Read the model definition and answer for the solid it produces. Units are mm, in the model's axes. A direction names the side the tool comes from. Round coordinates to 2 decimals unless told otherwise and drop trailing zeros. Order: outer loops, then holes, each group sorted by start corner. A loop starts at its lowest first (then second) coordinate and runs counter-clockwise, first axis right, second up. Notation, with made-up numbers: (-36.5, 58.25) -> (-12.5, 58.25) arc R19 cw to (-12.5, 70.25) -> close; hole circle Ø3 at (45, 37). An arc over 180 degrees is marked (long way). Answer as a JSON object with one key per item and string values. Group by question number.
Item 1: Section B-B, the plane y = -3 is taken. Write down the section's boundary in (x, z).
Item 2: Given P1, Ø8, axis at y = -0.5, z = 73, coming from the -X side; P2, Ø1.6, axis at x = -35, y = 2.5, coming from the +Z side; P3, Ø0.6, axis at x = -35.5, y = 3, coming from the -Z side, each flat-ended and moving along its own axis, determine where each tip first touches the part or whether it passes through.
Item 3: The mould has two halves that part along Z. Classify faces 4 (the flat face through (24.54, 7.54, 36.8)), 5 (the flat face through (-35, 0, 46)), 6 (the flat face through (33.5, 5, 44)), 7 (the cylindrical face through (-11.82, 7.535, 14.887)): pulls with the +Z half, pulls with the -Z half, needs draft (parallel to the pull), parting line crosses it, or undercut.
Item 4: Section A-A, the plane z = 52 is taken. Write down the section's boundary in (x, y).
Item 5: Section C-C, the plane z = 35.5 is taken. Write down the section's boundary in (x, y).
Item 6: Consider probe 1 along X at (y, z) = (8, -2.5); probe 2 along Z at (x, y) = (-28.5, 7.25); probe 3 along Z at (x, y) = (29, 4). Determine where each line is inside the solid, lowest interval first. Write a range as from..to.
Item 7: Section D-D, the plane z = -11 is taken. Write down the section's boundary in (x, y), plus the area to 3 significant figures.
Item 8: For faces 1 (the flat face through (0, 5, 2.5)), 2 (the flat face through (-30.44, 0.94, 88.3)), 3 (the flat face through (0, 2, -5)), determine the directions among +Z, -Z, +X, -X, +Y, -Y from which every point of the face is accessible in a straight line to the end or side of a thin tool.
from build123d import *

# Parameters (mm, degrees)
BOSS_EXTRUDE1_DEPTH = 10
FILLET2_R           = 30
SKETCH6_R           = 1
BOSS_EXTRUDE2_DEPTH = 5
SKETCH4_W           = 2
SKETCH4_H           = 1.5
CUT_EXTRUDE1_DEPTH  = 99.900202224
FILLET3_R           = 15
CUT_REVOLVE1_START  = -1
CUT_REVOLVE1_DEPTH  = 3.5
FILLET1_R           = 10
FILLET4_R           = 1
FILLET5_R           = 2
BOSS_EXTRUDE3_START = -10
BOSS_EXTRUDE3_DEPTH = 15
DELETEFACE1_DEPTH   = 11
FILLET6_R           = 3
FILLET7_R           = 3
BOSS_EXTRUDE4_START = -10
SKETCH11_W          = 10
SKETCH11_H          = 0.3
BOSS_EXTRUDE4_DEPTH = 8
FILLET8_R           = 0.3


with BuildPart() as part:
    # Sketch2 → Boss-Extrude1 (new body)
    with BuildSketch(Plane(origin=(0, 0, 0), x_dir=(1, 0, 0), z_dir=(0, 1, 0))):
        with BuildLine():
            Line((-15, 2.5), (-15, -2.5))
            Line((-15, -2.5), (15, -2.5))
            Line((15, -2.5), (15, 2.5))
            Line((15, 2.5), (-12, 2.5))
            ThreePointArc((-12, 2.5), (-36.874067112, 16.717067208), (-36.5, -11.93086969))
            Line((-36.5, -11.93086969), (-36.5, -66.907529531))
            ThreePointArc((-36.5, -66.907529531), (-34.28320825, -78.052094241), (-27.970319449, -87.5))
            Line((-27.970319449, -87.5), (-25.848999105, -85.378679656))
            ThreePointArc((-25.848999105, -85.378679656), (-31.511569653, -76.904043944), (-33.5, -66.907529531))
            Line((-33.5, -66.907529531), (-33.5, -10.039936204))
            ThreePointArc((-33.5, -10.039936204), (-36.074628704, 13.674748319), (-15, 2.5))
        make_face()
    boss_extrude1 = extrude(amount=BOSS_EXTRUDE1_DEPTH)

    # Mirror2: Boss-Extrude1 across plane
    add(boss_extrude1.mirror(Plane(origin=(0, 0, 0), x_dir=(0, 0, 1), z_dir=(1, 0, 0))))

    # Fillet2
    fillet2_edges = [part.edges().sort_by_distance(p)[0] for p in [
        (-36.5, 5, 11.93086969),
        (36.5, 5, 11.93086969),
    ]]
    fillet(fillet2_edges, radius=FILLET2_R)

    # Sketch6 → Boss-Extrude2 (add)
    # profile 1 of 2: a face of its own
    with BuildSketch(Plane(origin=(0, 10, 0), x_dir=(1, 0, 0), z_dir=(0, 1, 0))):
        with BuildLine():
            Line((-32.29175747, -29.0937848), (-16.524124365, -17.1403988))
            ThreePointArc((-16.524124365, -17.1403988), (-11.748018495, -14.869514069), (-6.462616651, -14.688870483))
            ThreePointArc((-6.462616651, -14.688870483), (-4.151991915, -13.057609213), (-5.783253184, -10.746984477))
            ThreePointArc((-5.783253184, -10.746984477), (-12.694932518, -10.983210705), (-18.940609425, -13.9528292))
            Line((-18.940609425, -13.9528292), (-34.70824253, -25.9062152))
            ThreePointArc((-34.70824253, -25.9062152), (-35.0937848, -28.70824253), (-32.29175747, -29.0937848))
        make_face()
        with Locations(Location((-6.122934918, -12.71792748, 0), (0, 0, 270))):
            Circle(SKETCH6_R, mode=Mode.SUBTRACT)
    # profile 2 of 2: a face of its own
    with BuildSketch(Plane(origin=(0, 10, 0), x_dir=(1, 0, 0), z_dir=(0, 1, 0))):
        with BuildLine():
            Line((32.29175747, -25.9062152), (16.524124365, -37.8596012))
            ThreePointArc((16.524124365, -37.8596012), (11.748018495, -40.130485931), (6.462616651, -40.311129517))
            ThreePointArc((6.462616651, -40.311129517), (4.151991915, -41.942390787), (5.783253184, -44.253015523))
            ThreePointArc((5.783253184, -44.253015523), (12.694932518, -44.016789295), (18.940609425, -41.0471708))
            Line((18.940609425, -41.0471708), (34.70824253, -29.0937848))
            ThreePointArc((34.70824253, -29.0937848), (35.0937848, -26.29175747), (32.29175747, -25.9062152))
        make_face()
        with Locations(Location((6.122934918, -42.28207252, 0), (0, 0, 270))):
            Circle(SKETCH6_R, mode=Mode.SUBTRACT)
    extrude(amount=-BOSS_EXTRUDE2_DEPTH)

    # Sketch4 → Cut-Extrude1 (cut, through all)
    with BuildSketch(Plane(origin=(0, 10, 0), x_dir=(1, 0, 0), z_dir=(0, 1, 0))):
        with BuildLine():
            Line((-13.2, 2.5), (-13.2, -2.5))
            Line((-13.2, -2.5), (-14.040055325, -2.5))
            ThreePointArc((-14.040055325, -2.5), (-43.588524672, 5.0350391), (-13.2, 2.5))
        make_face()
        with Locations((-35.5, -59.25)):
            Rectangle(SKETCH4_W, SKETCH4_H)
        with Locations((-35.5, -62.75)):
            Rectangle(SKETCH4_W, SKETCH4_H)
        with Locations((-35.5, -55.75)):
            Rectangle(SKETCH4_W, SKETCH4_H)
        with Locations((-35.5, -66.25)):
            Rectangle(SKETCH4_W, SKETCH4_H)
        with Locations((-35.5, -69.75)):
            Rectangle(SKETCH4_W, SKETCH4_H)
        with Locations((35.5, -69.75)):
            Rectangle(SKETCH4_W, SKETCH4_H)
        with Locations((35.5, -66.25)):
            Rectangle(SKETCH4_W, SKETCH4_H)
        with Locations((35.5, -62.75)):
            Rectangle(SKETCH4_W, SKETCH4_H)
        with Locations((35.5, -55.75)):
            Rectangle(SKETCH4_W, SKETCH4_H)
        with Locations((35.5, -59.25)):
            Rectangle(SKETCH4_W, SKETCH4_H)
        with BuildLine():
            Line((13.2, -2.5), (14.040055325, -2.5))
            ThreePointArc((14.040055325, -2.5), (43.588524672, 5.0350391), (13.2, 2.5))
            Line((13.2, 2.5), (13.2, -2.5))
        make_face()
    extrude(amount=-CUT_EXTRUDE1_DEPTH, mode=Mode.SUBTRACT)

    # Fillet3
    fillet3_edges = [part.edges().sort_by_distance(p)[0] for p in [
        (33.5, 5, 11.959944675),
        (-33.5, 5, 11.959944675),
    ]]
    fillet(fillet3_edges, radius=FILLET3_R)

    # Cut-Revolve1: read off the stored shape, not the designer's step
    # Cut-Revolve1 outline → Cut-Revolve1 (cut)
    with BuildSketch(Plane(origin=(0, 0, 0), x_dir=(1, 0, 0), z_dir=(0, 1, 0)).offset(CUT_REVOLVE1_START)):
        with BuildLine():
            ThreePointArc((-41.983870968, -7.00974362), (-39.626617248, -9.683939782), (-36.75, -11.789419162))
            Line((-36.75, -11.789419162), (-36.469117037, -11.3029156))
            ThreePointArc((-36.469117037, -11.3029156), (-37.473434742, -10.092280811), (-38.599009901, -8.993476368))
            ThreePointArc((-38.599009901, -8.993476368), (-34.807739235, 16.439240501), (-13.2, 2.5))
            Line((-13.2, 2.5), (-12, 2.5))
            ThreePointArc((-12, 2.5), (-33.488292745, 18.227903086), (-41.983870968, -7.00974362))
        make_face()
    cut_revolve1 = extrude(amount=CUT_REVOLVE1_DEPTH, mode=Mode.SUBTRACT)

    # Mirror3: Cut-Revolve1 across plane
    add(cut_revolve1.mirror(Plane(origin=(0, 0, 0), x_dir=(0, 0, 1), z_dir=(1, 0, 0))), mode=Mode.SUBTRACT)

    # Fillet1
    fillet1_edges = [part.edges().sort_by_distance(p)[0] for p in [
        (-12, 6.25, -2.5),
        (12, 6.25, -2.5),
    ]]
    fillet(fillet1_edges, radius=FILLET1_R)

    # Fillet4
    # the kernel refuses this fillet: 1 mm, written as the material it takes off along each edge
    with BuildSketch(Plane(origin=(41.983870968, -16.048184468, 7.00974362), x_dir=(-0.7225326531123375, 0, 0.6913367957706624), z_dir=(0, 1, 0))) as fillet4_piece_1:
        with BuildLine():
            CenterArc((6.528208905, 0.981393724), FILLET4_R, 113.353303502, 145.576812808)
            ThreePointArc((6.131809124, 1.899471723), (3.116855905, 0.785256492), (0, 0))
            ThreePointArc((0, 0), (3.168101381, 0.307003562), (6.336202761, 0))
        make_face()
    extrude(amount=18.548184468, mode=Mode.SUBTRACT)
    with BuildSketch(Plane(origin=(-41.983870968, -16.048184468, 7.00974362), x_dir=(0.7225326531123378, 0, 0.6913367957706622), z_dir=(0, 1, 0))) as fillet4_piece_2:
        with BuildLine():
            CenterArc((6.528208905, -0.981393724), FILLET4_R, 101.06988369, 145.576812808)
            ThreePointArc((6.131809124, -1.899471723), (3.116855905, -0.785256492), (0, 0))
            ThreePointArc((0, 0), (3.168101381, -0.307003562), (6.336202761, 0))
        make_face()
    extrude(amount=18.548184468, mode=Mode.SUBTRACT)

    # Fillet5
    fillet5_edges = [part.edges().sort_by_distance(p)[0] for p in [
        (-33.5, 7.5, 29.5),
        (-33.5, 7.5, 24.99025088),
        (33.5, 7.5, 25.5),
        (33.5, 7.5, 30.00974912),
    ]]
    fillet(fillet5_edges, radius=FILLET5_R)

    # Sketch8 → Boss-Extrude3 (add)
    with BuildSketch(Plane.XZ.offset(BOSS_EXTRUDE3_START)):
        with BuildLine():
            Line((-26.213914484, 95.605099549), (-31.869667291, 94.247080891))
            Line((-31.869667291, 94.247080891), (-27.783825698, 77.230738791))
            Line((-27.783825698, 77.230738791), (-22.128072891, 78.588757448))
            ThreePointArc((-22.128072891, 78.588757448), (-26.909659277, 86.439339828), (-26.213914484, 95.605099549))
        make_face()
    boss_extrude3 = extrude(amount=BOSS_EXTRUDE3_DEPTH)

    # Mirror4: Boss-Extrude3 across plane
    add(boss_extrude3.mirror(Plane(origin=(0, 0, 0), x_dir=(0, 0, 1), z_dir=(1, 0, 0))))

    # DeleteFace1: read off the stored shape, not the designer's step
    # DeleteFace1 outline → DeleteFace1 (cut)
    with BuildSketch(Plane(origin=(0, 0, 0), x_dir=(1, 0, 0), z_dir=(0, 1, 0))):
        with BuildLine():
            Line((25.848999105, -85.378679656), (26.909659277, -86.439339828))
            ThreePointArc((26.909659277, -86.439339828), (26.685366049, -85.610488056), (26.414012779, -84.795828548))
            ThreePointArc((26.414012779, -84.795828548), (26.133770133, -85.089449001), (25.848999105, -85.378679656))
        make_face()
        with BuildLine():
            Line((-26.909659277, -86.439339828), (-25.848999105, -85.378679656))
            ThreePointArc((-25.848999105, -85.378679656), (-26.133770133, -85.089449001), (-26.414012779, -84.795828548))
            ThreePointArc((-26.414012779, -84.795828548), (-26.685366049, -85.610488056), (-26.909659277, -86.439339828))
        make_face()
    extrude(amount=DELETEFACE1_DEPTH, mode=Mode.SUBTRACT)

    # Fillet6
    fillet6_edges = [part.edges().sort_by_distance(p)[0] for p in [
        (-31.869667291, 2.5, 94.247080891),
        (-29.774582906, 5, 85.521663663),
        (-27.783825698, 2.5, 77.230738791),
        (29.774582906, 5, 85.521663663),
        (27.783825698, 2.5, 77.230738791),
        (31.869667291, 2.5, 94.247080891),
    ]]
    fillet(fillet6_edges, radius=FILLET6_R)

    # Fillet7
    # the kernel refuses this fillet: 3 mm, written as the material it adds along each edge
    with BuildSketch(Plane(origin=(28.870158832, 10, 81.755000397), x_dir=(-0.4451552484524621, 0, -0.8954534073726151), z_dir=(0, -1, 0))) as fillet7_piece_1:
        with BuildLine():
            CenterArc((5.429938119, 2.554031947), FILLET7_R, 138.932760823, 99.425389741)
            Line((3.168120681, 4.524864735), (2.941938938, 4.721948013))
            ThreePointArc((2.941938938, 4.721948013), (1.218371107, 2.518472645), (-0.262566045, 0.145117443))
            Line((-0.262566045, 0.145117443), (0.067135427, -0.292391577))
            ThreePointArc((0.067135427, -0.292391577), (1.678072021, 0.077492249), (3.698732127, -0.255403195))
            Line((3.698732127, -0.255403195), (3.85611449, 0))
        make_face()
    extrude(amount=10)
    with BuildSketch(Plane(origin=(-28.870158832, 10, 81.755000397), x_dir=(-0.47821106545327013, 0, -0.8782449412766623), z_dir=(0, -1, 0))) as fillet7_piece_2:
        with BuildLine():
            CenterArc((5.206526078, 2.983185104), FILLET7_R, 176.643750304, 99.425389741)
            Line((2.21167161, 3.158817444), (1.912186163, 3.176380678))
            ThreePointArc((1.912186163, 3.176380678), (1.025936374, 1.330182436), (-0.201013248, 0.222696372))
            Line((-0.201013248, 0.222696372), (-0.031718549, -0.29831851))
            ThreePointArc((-0.031718549, -0.29831851), (2.761855785, -0.446413754), (5.55543012, -0.29831851))
            Line((5.55543012, -0.29831851), (5.523711571, 0))
        make_face()
    extrude(amount=10)

    # Sketch11 → Boss-Extrude4 (add)
    with BuildSketch(Plane.XZ.offset(BOSS_EXTRUDE4_START)):
        Polygon((-7.309401077, -6.8), (7.309401077, -6.8), (5, -2.8), (-5, -2.8), align=None)
        with Locations((0, -2.65)):
            Rectangle(SKETCH11_W, SKETCH11_H)
    extrude(amount=BOSS_EXTRUDE4_DEPTH)

    # Fillet8
    fillet8_edges = [part.edges().sort_by_distance(p)[0] for p in [
        (-7.309401077, 6, -6.8),
        (7.309401077, 6, -6.8),
    ]]
    fillet(fillet8_edges, radius=FILLET8_R)


solid = part.part
Values found:
{
 "1": {"outline": "(-31.17, 91.33) -> (-28.48, 80.15) arc R3 ccw to (-24.87, 77.93) -> (-22.13, 78.59) arc R15 cw to (-26.21, 95.61) -> (-28.95, 94.95) arc R3 ccw to start; (22.13, 78.59) -> (24.87, 77.93) arc R3 ccw to (28.48, 80.15) -> (31.17, 91.33) arc R3 ccw to (28.95, 94.95) -> (26.21, 95.61) arc R15 cw to start"},
 "2": {"P1": "x = -36.28", "P2": "z = 78.25", "P3": "z = -17.58"},
 "3": {"face 4": "undercut", "face 5": "needs draft", "face 6": "undercut", "face 7": "pulls with the +Z half"},
 "4": {"outline": "(-36.5, 0) -> (-33.5, 0) -> (-33.5, 10) -> (-36.5, 10) -> close; (33.5, 0) -> (36.5, 0) -> (36.5, 10) -> (33.5, 10) -> close"},
 "5": {"outline": "(-36.5, 0) -> (-33.5, 0) -> (-33.5, 10) -> (-36.5, 10) -> close; (19.64, 5) -> (26.26, 5) -> (26.26, 10) -> (19.64, 10) -> close; (33.5, 0) -> (36.5, 0) -> (36.5, 10) -> (33.5, 10) -> close"},
 "6": {"probe 1": "-45..-43.8, -13.2..13.2, 43.8..45", "probe 2": "-19..-17.8, 21.2..26.22, 78.75..95.06", "probe 3": "-18.99..-17.79, 78.74..94.94"},
 "7": {"outline": "(-42.64, 2.5) -> (-41.22, 2.5) -> (-41.22, 10) -> (-42.64, 10) -> close; (-15.78, 2.5) -> (-14.36, 2.5) -> (-14.36, 10) -> (-15.78, 10) -> close; (14.36, 2.5) -> (15.78, 2.5) -> (15.78, 10) -> (14.36, 10) -> close; (41.22, 2.5) -> (42.64, 2.5) -> (42.64, 10) -> (41.22, 10) -> close", "area": "42.6 mm2"},
 "8": {"face 1": "+Y, -Y", "face 2": "-X, -Y", "face 3": "-Z, +X, -X, -Y"}
}
